Part model, mm, in its own coordinate system. Face numbers are marked on the shaded views. A direction names the side the tool comes from. Round coordinates to 2 decimals unless told otherwise and drop trailing zeros. Order: outer loops, then holes, each group sorted by start corner. A loop starts at its lowest first (then second) coordinate and runs counter-clockwise, first axis right, second up. Notation, with made-up numbers: (39, 41.5) - (51, 41.5) arc R8 cw to (51, 56.5) - close; hole circle Ø11 at (-28, -6.75). An arc over 180 degrees is marked (long way). Return JSON: item names as keys, results as strings. Group by question number.
Item 1: Saw through at D-D on y = -9.5. List the corners of the cut face in (x, z).
Item 2: Saw through at A-A on y = -25. List the corners of the cut face in (x, z).
Item 3: Drop flat-ended pins along their axis: pin 1 (1 mm diameter, centred on x = -6.5, y = -11, fed in from -Z); pin 2 (4 mm diameter, centred on x = 3, y = -20, fed in from +Z); pin 3 (1.1 mm diameter, centred on y = -19, z = 1, fed in from -X); pin 4 (2.5 mm diameter, centred on x = 1.99, y = -25, fed in from +Z). Give the stop position or say it passes through.
Item 4: Saw through at B-B on z = 1. List the corners of the cut face in (x, y).
Item 5: Probe probe 1 along X at (y, z) = (-5, 0.55); probe 2 along Y at (x, z) = (3.5, 2.25); probe 3 along X at (y, z) = (-11.5, 4.25). List the from-to ranges inside material, lowest first.
Item 6: Saw through at C-C on x = -5. List the corners of the cut face in (y, z), and give its area (3 significant figures).
Item 7: Tool access for the marked faces 1, 2 and 3: list every direction of +Z, -Z, +X, -X, +Y, -Y with a clear straight run to the whole face (end or side of a thin tool).
Item 8: Two-plate mould, pull along Y, no slides. Class the marked faces 4, 5 and 6: released by +Y, released by -Y, zero draft, split by the parting line, or undercut.
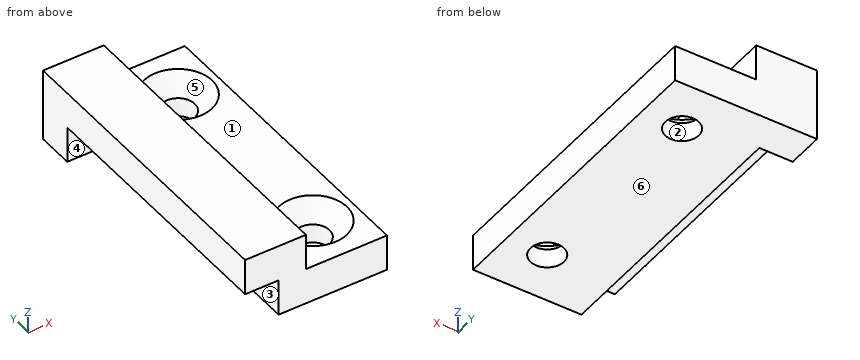
```python
from build123d import *

# Parameters (mm, degrees)
F1_DEPTH       = 30
F3_D           = 3.3
F3_CSINK_D     = 6.72
F3_CSINK_ANGLE = 90
F4_W           = 3.6
F4_H           = 3.6
F5_DEPTH       = 3.3


with BuildPart() as f1:
    # F0 (on Front) → F1 (new body)
    with BuildSketch(Plane.XZ):
        Polygon((-4.7134831967, 0), (5.9865168033, 0), (5.9865168033, 3.6), (-2.0134831967, 3.6), (-2.0134831967, 7.2), (-8.0134831967, 7.2), (-8.0134831967, 3.6), (-4.7134831967, 3.6), align=None)
    extrude(amount=F1_DEPTH)

    # F3 (through all)
    with Locations(Plane.XY.offset(3.6)):
        with Locations((1.9865168033, -5), (1.9865168033, -25)):
            CounterSinkHole(F3_D / 2, F3_CSINK_D / 2, counter_sink_angle=F3_CSINK_ANGLE)

    # F4 (on face) → F5 (join, through all)
    with BuildSketch(Plane(origin=(-4.7134831967, 0, 0), x_dir=(0, -1, 0), z_dir=(-1, 0, 0))):
        with Locations((1.8, 1.8)):
            Rectangle(F4_W, F4_H)
    extrude(amount=F5_DEPTH)


solid = f1.part
```
Filled in:
{
 "1": {"outline": "(-8.01, 3.6) - (-4.71, 3.6) - (-4.71, 0) - (5.99, 0) - (5.99, 3.6) - (-2.01, 3.6) - (-2.01, 7.2) - (-8.01, 7.2) - close"},
 "2": {"outline": "(-8.01, 3.6) - (-4.71, 3.6) - (-4.71, 0) - (0.34, 0) - (0.34, 1.89) - (-1.37, 3.6) - (-2.01, 3.6) - (-2.01, 7.2) - (-8.01, 7.2) - close; (3.64, 0) - (5.99, 0) - (5.99, 3.6) - (5.35, 3.6) - (3.64, 1.89) - close"},
 "3": {"pin 1": "stops at z = 3.6", "pin 2": "stops at z = 3.6", "pin 3": "stops at x = -4.71", "pin 4": "passes through"},
 "4": {"outline": "(-8.01, -3.6) - (-4.71, -3.6) - (-4.71, -30) - (5.99, -30) - (5.99, 0) - (-8.01, 0) - close; hole circle Ø3.3 at (1.99, -25); hole circle Ø3.3 at (1.99, -5)"},
 "5": {"probe 1": "x = -4.71 to 0.34, 3.64 to 5.99", "probe 2": "y = -30 to -26.32, -23.68 to -6.32, -3.68 to 0", "probe 3": "x = -8.01 to -2.01"},
 "6": {"outline": "(-30, 3.6) - (-3.6, 3.6) - (-3.6, 0) - (0, 0) - (0, 7.2) - (-30, 7.2) - close", "area": "121 mm^2"},
 "7": {"face 1": "+Z, +X, +Y, -Y", "face 2": "+Z, -Z", "face 3": "-Z, -X, -Y"},
 "8": {"face 4": "released by -Y", "face 5": "undercut", "face 6": "zero draft"}
}
